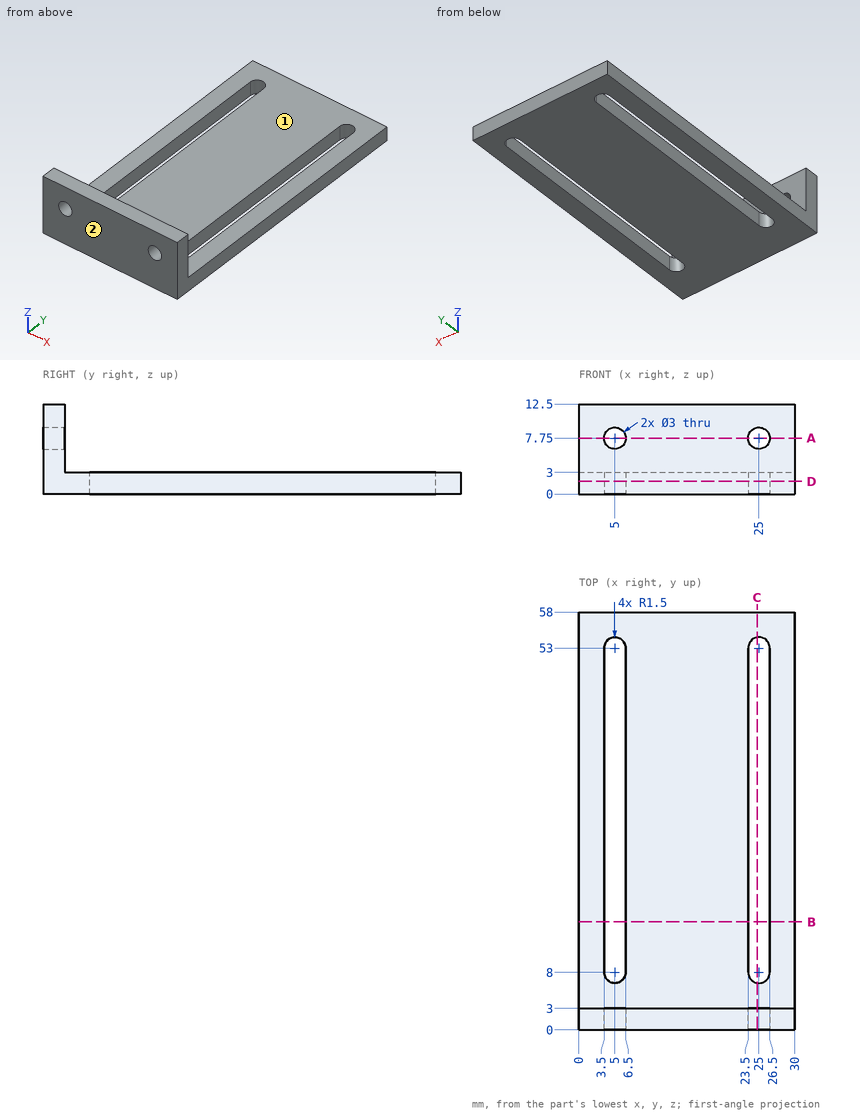
Input: dimensioned drawing with shaded views. Units: mm. Origin: part minimum x, y, z. A direction names the side the tool comes from. Coordinates: 2 decimals unless noted, no trailing zeros. Order: outer loops, then holes, each group sorted by start corner. A loop starts at its lowest first (then second) coordinate and runs counter-clockwise, first axis right, second up. Notation, with made-up numbers: (7, 80.5) - (13, 80.5) arc R29 cw to (13, 113.5) - close; hole circle Ø10 at (6.25, 11.25). An arc over 180 degrees is marked (long way). One line per item, written item: value.
1) Cut plane A-A on z = 7.75. Output: boundary loops of the cut face in (x, y).
Computed values:
outline: (0, 0) - (3.5, 0) - (3.5, 3) - (0, 3) - close; (6.5, 0) - (23.5, 0) - (23.5, 3) - (6.5, 3) - close; (26.5, 0) - (30, 0) - (30, 3) - (26.5, 3) - close
2) Cut plane D-D on z = 1.75. Output: boundary loops of the cut face in (x, y), plus the area to 3 significant figures.
Computed values:
outline: (0, 0) - (30, 0) - (30, 58) - (0, 58) - close; hole (3.5, 8) arc R1.5 ccw to (6.5, 8) - (6.5, 53) arc R1.5 ccw to (3.5, 53) - close; hole (23.5, 8) arc R1.5 ccw to (26.5, 8) - (26.5, 53) arc R1.5 ccw to (23.5, 53) - close
area: 1,460 mm^2
3) Reachability of the marked faces 1 and 2 from +Z, -Z, +X, -X, +Y, -Y: full face, straight path, thin tool, end or side. Return the list, or none.
Computed values:
face 1: +Z, +X, -X, +Y
face 2: +Z, -Z, +X, -X, -Y
4) Ray query, line 1 (X direction, y = 1.35, z = 7.75); line 2 (Z direction, x = 25, y = 1.7); line 3 (Y direction, x = 19.75, z = 4). Return the intervals inside material, ascending. Write a range as [from, to].
Computed values:
line 1: x = [0, 3.5], [6.5, 23.5], [26.5, 30]
line 2: z = [0, 6.25], [9.25, 12.5]
line 3: y = [0, 3]
5) Cut plane C-C on x = 24.75. Output: boundary loops of the cut face in (y, z).
Computed values:
outline: (0, 0) - (6.52, 0) - (6.52, 3) - (3, 3) - (3, 6.27) - (0, 6.27) - close; (0, 9.23) - (3, 9.23) - (3, 12.5) - (0, 12.5) - close; (54.48, 0) - (58, 0) - (58, 3) - (54.48, 3) - close
6) Contact query for flat-ended pins moving along their axis: pin 1 (5 mm diameter, centred on x = 5, z = 7.75, fed in from +Y); pin 2 (4 mm diameter, centred on y = 48.5, z = 6.5, fed in from +X); pin 3 (10 mm diameter, centred on x = 10, y = 11.5, fed in from +Z). Output: stop coordinate, or through.
Computed values:
pin 1: stops at y = 3
pin 2: passes through
pin 3: stops at z = 3
